Read the model definition and answer for the solid it produces. Units are mm, in the model's axes. A direction names the side the tool comes from. Coordinates: 2 decimals unless noted, no trailing zeros. Loops run counter-clockwise (first coordinate to the right, second up) from the corner with the lowest first, then second, coordinate; pieces in that order, holes last. Notation, with made-up numbers: (13.25, 3.5) - (67.25, 3.5) arc R18 cw to (67.25, 21.5) - close; hole circle Ø11 at (-18, 42). An arc over 180 degrees is marked (long way). One line per item, written item: value. Start each with the question number.
Autodesk Inventor part; units mm, degrees
ref_plane "YZ Plane" through (0, 0, 0) normal (1, 0, 0) x (0, 1, 0)
ref_plane "XZ Plane" through (0, 0, 0) normal (0, 1, 0) x (-1, 0, 0)
ref_plane "XY Plane" through (0, 0, 0) normal (0, 0, 1) x (1, 0, 0)
sketch "Sketch1" plane through (0, 0, 0) normal (0, 0, 1) x (1, 0, 0)
  line L0 (-64, 50) -> (64, 50)
  line L1 (64, 50) -> (64, 0)
  line L2 (64, 0) -> (-64, 0)
  line L3 (-64, 0) -> (-64, 50)
  line L4 (-25, 0) -> (25, 0)
  line L5 (25, 0) -> (25, -2)
  line L6 (25, -2) -> (-25, -2)
  line L7 (-25, -2) -> (-25, 0)
  point P0 (0, 0)
  point P1 (0, 0)
  dimension "d0" = 50
  dimension "d1" = 128
  dimension "d2" = 2
  dimension "d3" = 50
extrude "Extrusion1" add sketch "Sketch1" along normal mid plane 2
sketch "Sketch2" plane through (0, 0, 1) normal (0, 0, 1) x (1, 0, 0)
  line L0 (-37.004, 19.1647) -> (37.8795, 15.001)
  line L1 (37.8795, 15.001) -> (37.8795, 6.0072)
  line L2 (37.8795, 6.0072) -> (-37.004, 10.1709)
  line L3 (-37.004, 10.1709) -> (-37.004, 19.1647)
  line L4 (41.9117, 3.4023) -> (41.9117, 13.1647)
  line L5 (-41.259, 17.7892) -> (-41.259, 8.0268)
  point P0 (0, 0)
sketch "Sketch3" plane through (0, 0, 1) normal (0, 0, 1) x (1, 0, 0)
  line L0 (-41.259, 17.7892) -> (-41.259, 8.0268) construction
  line L1 (37.8795, 6.0072) -> (-37.004, 10.1709) construction
  line L2 (41.9117, 3.4023) -> (41.9117, 13.1647) construction
  line L3 (-41.259, 10.4075) -> (41.9117, 5.783)
  line L4 (-41.259, 10.4075) -> (-41.259, 0)
  line L5 (-41.259, 0) -> (-91.259, 0)
  line L6 (-91.259, 0) -> (-91.259, 60)
  line L7 (-91.259, 60) -> (91.9117, 60)
  line L8 (91.9117, 60) -> (91.9117, 0)
  line L9 (91.9117, 0) -> (41.9117, 0)
  line L10 (41.9117, 0) -> (41.9117, 5.783)
  point P0 (0, 0)
  dimension "d6" = 50
  dimension "d7" = 50
  dimension "d8" = 60
extrude "Extrusion2" cut sketch "Sketch3" against normal through all
sketch "Sketch4" plane through (0, 0, 1) normal (0, 0, 1) x (1, 0, 0)
  line L0 (-37, 0) -> (-37, 9.5832)
  line L1 (-35, 0) -> (-37, 0)
  line L2 (-35, 9.5832) -> (-35, 0)
  line L3 (-35, 9.5832) -> (-37, 9.5832)
  line L4 (36, 0) -> (36, 5.3914)
  line L5 (38, 0) -> (36, 0)
  line L6 (38, 5.3914) -> (38, 0)
  line L7 (38, 5.3914) -> (36, 5.3914)
  point P0 (0, 0)
sketch "Sketch5" plane through (0, 0, 1) normal (0, 0, 1) x (1, 0, 0)
  line L0 (-37, 0) -> (-37, 9.5832) construction
  line L1 (-35, 9.5832) -> (-35, 0) construction
  line L2 (36, 0) -> (36, 5.3914) construction
  line L3 (38, 5.3914) -> (38, 0) construction
  line L4 (-37, 4) -> (-35, 4)
  line L5 (-35, 4) -> (-35, 0)
  line L6 (-35, 0) -> (-37, 0)
  line L7 (-37, 0) -> (-37, 4)
  line L8 (38, 4) -> (36, 4)
  line L9 (36, 4) -> (36, 0)
  line L10 (36, 0) -> (38, 0)
  line L11 (38, 0) -> (38, 4)
  point P0 (0, 0)
  dimension "d11" = 4
  dimension "d12" = 4
extrude "Extrusion3" cut sketch "Sketch5" against normal through all
properties part number "angle_plate_short_short"
1) Straight lines are drawn through the part: L1, parallel to X at y = 3, z = -0.7; L2, parallel to X at y = -0.75, z = 0.25; L3, parallel to Y at x = 33, z = -0.3. For each, find the intervals that lie inside material, in ascending order.
2) Flat-ended cylindrical pins translate along their axes: P1, Ø0.6, axis at x = 41, z = 0.5, coming from the -Y side; P2, Ø1, axis at x = 9, z = -0.5, coming from the +Y side. Find the tip coordinate at first contact, or state that the pin passes through.
3) For faces 4 (the flat face through (-41.259, 5, 0)), 5 (the flat face through (-36, 4, 0)), 6 (the flat face through (-30, 0, 0)), 7 (the flat face through (40, 0, 0)), determine the directions among +Z, -Z, +X, -X, +Y, -Y from which every point of the face is accessible in a straight line to the end or side of a thin tool.
4) Section C-C, the plane x = 26 is taken. Determine the outline of the cut face in (y, z), and give its area (3 significant figures).
5) Determine the mould class of faces 1 (the flat face through (0, -2, 0)), 2 (the flat face through (-35, 2, 0)), 3 (the flat face through (25, -1, 0)) for opening direction X: released by +X, released by -X, zero draft, split by the parting line, or undercut.
6) Section B-B, the plane z = -0.45 is taken. Determine the outline of the cut face in (x, y).
7) Section D-D, the plane y = 9 is taken. Determine the outline of the cut face in (x, z), and give its area (3 significant figures).
8) Section A-A, the plane y = 1 is taken. Determine the outline of the cut face in (x, z).
Answer below:
1. L1: -41.26 to -37, -35 to 36, 38 to 41.91
1. L2: -25 to 25
1. L3: 0 to 6.28
2. P1: y = 0
2. P2: y = 7.64
3. face 4: +Z, -Z, -X, +Y, -Y
3. face 5: +Z, -Z, -Y
3. face 6: +Z, -Z, -X, -Y
3. face 7: +Z, -Z, +X, -Y
4. outline: (0, -1) - (6.67, -1) - (6.67, 1) - (0, 1) - close
4. area: 13.3 mm2
5. face 1: zero draft
5. face 2: undercut
5. face 3: released by +X
6. outline: (-41.26, 0) - (-37, 0) - (-37, 4) - (-35, 4) - (-35, 0) - (-25, 0) - (-25, -2) - (25, -2) - (25, 0) - (36, 0) - (36, 4) - (38, 4) - (38, 0) - (41.91, 0) - (41.91, 5.78) - (-41.26, 10.41) - close
7. outline: (-41.26, -1) - (-15.95, -1) - (-15.95, 1) - (-41.26, 1) - close
7. area: 50.6 mm2
8. outline: (-41.26, -1) - (-37, -1) - (-37, 1) - (-41.26, 1) - close; (-35, -1) - (36, -1) - (36, 1) - (-35, 1) - close; (38, -1) - (41.91, -1) - (41.91, 1) - (38, 1) - close
